The listing builds one solid part. Answer for the finished solid, in the listing's coordinates (mm). Give positions to 0.01 mm unless a question says otherwise; leave off trailing zeros. Order: outer loops, then holes, each group sorted by start corner. A loop starts at its lowest first (then second) coordinate and runs counter-clockwise, first axis right, second up. Notation, with made-up numbers: (7, 45.25) - (54, 45.25) arc R16 ccw to (54, 56.25) - close; hole circle Ø11 at (38, -6). An arc over 180 degrees is marked (long way). Use a Markdown table: item, result. Add a question column.
1) Find section B-B, the plane z = -57. Determine the outline of the cut face in (x, y), plus the area to 3 significant figures.
2) Find section C-C, the plane y = 1.3. State how many separate pieces and enclosed holes the cut face has, plus the area to 3 significant figures.
3) Straight lines are drawn through the part: line 1 (X direction, y = 2.3, z = -24); line 2 (Z direction, x = -80, y = 3.9) (3 decimals); line 3 (Z direction, x = -87, y = 2.4). For each, find the intervals that lie inside material, in ascending order.
4) Find section A-A, the plane x = -45. Determine the outline of the cut face in (y, z).
5) Flat-ended cylindrical pins translate along their axes: pin 1 (2 mm diameter, centred on y = 3, z = 26, fed in from +X); pin 2 (1.3 mm diameter, centred on y = 2.5, z = 20, fed in from -X). Find the tip coordinate at first contact, or state that the pin passes through.
from build123d import *

# Parameters (mm, degrees)
SKETCH1_W            = 220
SKETCH1_H            = 220
SQUARE_DEPTH         = 4.5
SKETCH2_R            = 1.55
LM8UU_HOLDERS_DEPTH  = 156.628564216
SKETCH3_R            = 1.55
DEFAULTBELT_DEPTH    = 156.628564216
BELTOPTIONS_DEPTH    = 156.628564216
SKETCH5_OUTSIDE_W    = 284.232
SKETCH5_OUTSIDE_H    = 284.232
SHAPING_DEPTH        = 10
SKETCH6_R            = 1.55
CUT_EXTRUDE5_DEPTH   = 156.628564216
SKETCH7_W            = 11.5
SKETCH7_H            = 24.25
CUT_EXTRUDE6_DEPTH   = 156.628564216
SKETCH8_R            = 1.55
ENDSTOPTRIGGER_DEPTH = 156.628564216
LPATTERN1_COUNT      = 2
LPATTERN1_PITCH      = 30


with BuildPart() as part:
    # Sketch1 → Square (new body)
    with BuildSketch(Plane(origin=(0, 0, 0), x_dir=(1, 0, 0), z_dir=(0, 1, 0))):
        Rectangle(SKETCH1_W, SKETCH1_H)
    extrude(amount=SQUARE_DEPTH)

    # Sketch2 → LM8UU-Holders (cut, through all)
    with BuildSketch(Plane(origin=(0, 4.5, 0), x_dir=(1, 0, 0), z_dir=(0, 1, 0))):
        with Locations(Location((-87, 22, 0), (0, 0, 270))):
            Circle(SKETCH2_R)
        with Locations(Location((-87, 38, 0), (0, 0, 270))):
            Circle(SKETCH2_R)
        with Locations(Location((-63, 38, 0), (0, 0, 270))):
            Circle(SKETCH2_R)
        with Locations(Location((-63, 22, 0), (0, 0, 270))):
            Circle(SKETCH2_R)
        with Locations(Location((63, 22, 0), (0, 0, 270))):
            Circle(SKETCH2_R)
        with Locations(Location((63, 38, 0), (0, 0, 270))):
            Circle(SKETCH2_R)
        with Locations(Location((87, 38, 0), (0, 0, 270))):
            Circle(SKETCH2_R)
        with Locations(Location((87, 22, 0), (0, 0, 270))):
            Circle(SKETCH2_R)
        with Locations(Location((-87, -38, 0), (0, 0, 270))):
            Circle(SKETCH2_R)
        with Locations(Location((-87, -22, 0), (0, 0, 270))):
            Circle(SKETCH2_R)
        with Locations(Location((-63, -22, 0), (0, 0, 270))):
            Circle(SKETCH2_R)
        with Locations(Location((-63, -38, 0), (0, 0, 270))):
            Circle(SKETCH2_R)
        with Locations(Location((63, -38, 0), (0, 0, 270))):
            Circle(SKETCH2_R)
        with Locations(Location((63, -22, 0), (0, 0, 270))):
            Circle(SKETCH2_R)
        with Locations(Location((87, -22, 0), (0, 0, 270))):
            Circle(SKETCH2_R)
        with Locations(Location((87, -38, 0), (0, 0, 270))):
            Circle(SKETCH2_R)
    extrude(amount=-LM8UU_HOLDERS_DEPTH, mode=Mode.SUBTRACT)

    # Sketch3 → DefaultBelt (cut, through all)
    with BuildSketch(Plane(origin=(0, 4.5, 0), x_dir=(1, 0, 0), z_dir=(0, 1, 0))):
        with Locations(Location((-15, -30, 0), (0, 0, 270))):
            Circle(SKETCH3_R)
        with Locations(Location((15, -30, 0), (0, 0, 90))):
            Circle(SKETCH3_R)
        with Locations(Location((15, 0, 0), (0, 0, 270))):
            Circle(SKETCH3_R)
        with Locations(Location((-15, 0, 0), (0, 0, 90))):
            Circle(SKETCH3_R)
    defaultbelt = extrude(amount=-DEFAULTBELT_DEPTH, mode=Mode.SUBTRACT)

    # Sketch4 → BeltOptions (cut, through all)
    with BuildSketch(Plane(origin=(0, 4.5, 0), x_dir=(1, 0, 0), z_dir=(0, 1, 0))):
        with BuildLine():
            ThreePointArc((-0.916515139, 6.25), (0, 3.45), (0.916515139, 6.25))
            ThreePointArc((0.916515139, 6.25), (0, 9.05), (-0.916515139, 6.25))
        make_face()
        with BuildLine():
            ThreePointArc((0.916515139, -36.25), (0, -39.05), (-0.916515139, -36.25))
            ThreePointArc((-0.916515139, -36.25), (0, -33.45), (0.916515139, -36.25))
        make_face()
    extrude(amount=-BELTOPTIONS_DEPTH, mode=Mode.SUBTRACT)

    # Sketch5 outside → Shaping (cut)
    with BuildSketch(Plane(origin=(0, 4.5, 0), x_dir=(1, 0, 0), z_dir=(0, 1, 0))):
        Rectangle(SKETCH5_OUTSIDE_W, SKETCH5_OUTSIDE_H)
        Polygon((-110, 110), (-110, 80), (-95, 65), (-95, -65), (-110, -80), (-110, -110), (-80, -110), (-65, -95), (65, -95), (80, -110), (110, -110), (110, -80), (95, -65), (95, 65), (110, 80), (110, 110), (80, 110), (65, 95), (-65, 95), (-80, 110), align=None, mode=Mode.SUBTRACT)
    extrude(amount=-SHAPING_DEPTH, mode=Mode.SUBTRACT)

    # Sketch6 → Cut-Extrude5 (cut, through all)
    with BuildSketch(Plane(origin=(0, 4.5, 0), x_dir=(1, 0, 0), z_dir=(0, 1, 0))):
        with Locations(Location((-104.5, 104.5, 0), (0, 0, 270))):
            Circle(SKETCH6_R)
        with Locations(Location((104.5, 104.5, 0), (0, 0, 90))):
            Circle(SKETCH6_R)
        with Locations(Location((104.5, -104.5, 0), (0, 0, 270))):
            Circle(SKETCH6_R)
        with Locations(Location((-104.5, -104.5, 0), (0, 0, 90))):
            Circle(SKETCH6_R)
    extrude(amount=-CUT_EXTRUDE5_DEPTH, mode=Mode.SUBTRACT)

    # Sketch7 → Cut-Extrude6 (cut, through all)
    with BuildSketch(Plane(origin=(0, 4.5, 0), x_dir=(1, 0, 0), z_dir=(0, 1, 0))):
        with Locations((-75, 30)):
            Rectangle(SKETCH7_W, SKETCH7_H)
        with Locations((-75, -30)):
            Rectangle(SKETCH7_W, SKETCH7_H)
        with Locations((75, -30)):
            Rectangle(SKETCH7_W, SKETCH7_H)
        with Locations((75, 30)):
            Rectangle(SKETCH7_W, SKETCH7_H)
    extrude(amount=-CUT_EXTRUDE6_DEPTH, mode=Mode.SUBTRACT)

    # Sketch8 → EndstopTrigger (cut, through all)
    with BuildSketch(Plane(origin=(0, 4.5, 0), x_dir=(1, 0, 0), z_dir=(0, 1, 0))):
        with Locations(Location((-33.45, 45, 0), (0, 0, 270))):
            Circle(SKETCH8_R)
        with Locations(Location((-33.45, 40, 0), (0, 0, 270))):
            Circle(SKETCH8_R)
        with Locations(Location((-33.45, 35, 0), (0, 0, 270))):
            Circle(SKETCH8_R)
        with Locations(Location((-33.45, 30, 0), (0, 0, 270))):
            Circle(SKETCH8_R)
    extrude(amount=-ENDSTOPTRIGGER_DEPTH, mode=Mode.SUBTRACT)

    # LPattern1: DefaultBelt ×2
    with Locations(*[(0, 0, -i * LPATTERN1_PITCH) for i in range(1, LPATTERN1_COUNT)]):
        add(defaultbelt, mode=Mode.SUBTRACT)


solid = part.part
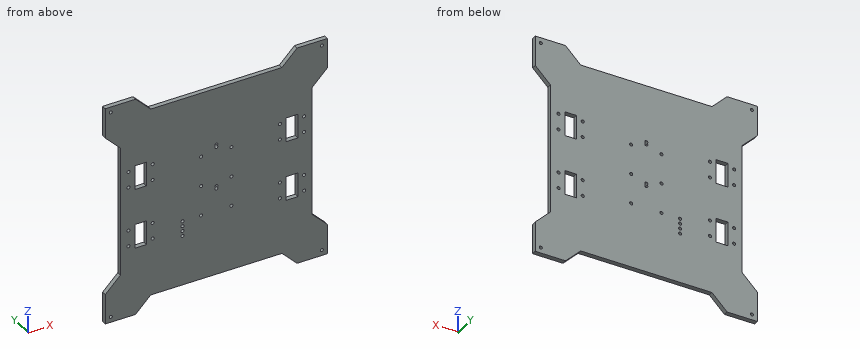
The answers:
| question | item | result |
|---|---|---|
| 1 | outline | (-95, 0) - (95, 0) - (95, 4.5) - (-95, 4.5) - close |
| 1 | area | 855 mm2 |
| 2 | separate pieces | 1 |
| 2 | enclosed holes | 36 |
| 2 | area | 38,300 mm2 |
| 3 | line 1 | -95 to -80.75, -69.25 to 69.25, 80.75 to 95 |
| 3 | line 2 | -110 to -42.125, -17.875 to 17.875, 42.125 to 110 |
| 3 | line 3 | -110 to -39.55, -36.45 to -23.55, -20.45 to 20.45, 23.55 to 36.45, 39.55 to 110 |
| 4 | outline | (0, -95) - (4.5, -95) - (4.5, 95) - (0, 95) - close |
| 5 | pin 1 | x = 95 |
| 5 | pin 2 | x = -95 |
